Source: CAD feature listing. Evaluate the final solid. Frame: model axes, mm. A direction names the side the tool comes from. Coordinates: 2 decimals unless noted, no trailing zeros. Order: outer loops, then holes, each group sorted by start corner. A loop starts at its lowest first (then second) coordinate and runs counter-clockwise, first axis right, second up. Notation, with made-up numbers: (76, 65.25) -> (83, 65.25) arc R6 ccw to (83, 75.25) -> close; hole circle Ø6 at (-17, 79.5). An arc over 180 degrees is marked (long way). Put each result on its own line as item: value.
from build123d import *

# Parameters (mm, degrees)
EXTRUDE_START            = 8.875
SKETCH1_R                = 7.5
SKETCH1_R_2              = 3
EXTRUDE_KNOB_DEPTH       = 16.5
EXTRUDE_START_2          = 25.375
SKETCH1_3_R              = 3
EXTRUDE_KNOB_INNER_DEPTH = 1
CHAMFER_KNOB_SIZE        = 0.5


with BuildPart() as part:
    # Sketch1 → extrude knob (new body)
    with BuildSketch(Plane.XY.offset(EXTRUDE_START)):
        with Locations((6.776307172, 8.001648034)):
            Circle(SKETCH1_R)
        with Locations((6.776307172, 8.001648034)):
            Circle(SKETCH1_R_2, mode=Mode.SUBTRACT)
    extrude(amount=EXTRUDE_KNOB_DEPTH)

    # Sketch1<3> → extrude knob inner (add)
    with BuildSketch(Plane.XY.offset(EXTRUDE_START_2)):
        with Locations((6.776307172, 8.001648034)):
            Circle(SKETCH1_3_R)
    extrude(amount=-EXTRUDE_KNOB_INNER_DEPTH)

    # chamfer knob
    chamfer_knob_edges = [part.edges().sort_by_distance(p)[0] for p in [
        (-0.723692828, 8.001648034, 25.375),
    ]]
    chamfer(chamfer_knob_edges, length=CHAMFER_KNOB_SIZE)


solid = part.part
1. Set-up query: faces 1 (the flat face through (10, 8, 8.875)), 2 (the cylindrical face through (6.386, 10.976, 16.516)). Return all of +Z, -Z, +X, -X, +Y, -Y with unobstructed straight access to the full face (end or side cutting, diameter ignored); none if empty.
Numbers:
face 1: -Z, +X, -X, +Y, -Y
face 2: -Z
2. First-contact query: pin 1 (6.5 mm diameter, centred on x = 6, y = 7.5, fed in from -Z) (3 decimals); pin 2 (1.5 mm diameter, centred on x = 4, z = 19.5, fed in from +Y); pin 3 (1 mm diameter, centred on x = 8, z = 16.5, fed in from -Y); pin 4 (6 mm diameter, centred on x = 11, z = 13.5, fed in from +Y). Flat tips, straight axial feed; report the tip coordinate or a pass-through.
Numbers:
pin 1: stops at z = 8.875
pin 2: stops at y = 15.22
pin 3: stops at y = 0.54
pin 4: stops at y = 15.4
3. Cut plane A-A on z = 21.5. Output: boundary loops of the cut face in (x, y).
Numbers:
outline: circle Ø15 at (6.78, 8); hole circle Ø6 at (6.78, 8)
4. Pull-direction query (Y, two-part tool) for faces 3 (the flat face through (7, 8, 25.375)), 4 (the flat face through (7, 8, 24.375)), 5 (the cylindrical face through (1.25, 13.07, 16.76)); classes: pulls with the +Y half, pulls with the -Y half, needs draft (parallel to the pull), parting line crosses it, or undercut.
Numbers:
face 3: needs draft
face 4: undercut
face 5: parting line crosses it
5. Ray query, line 1 along X through (y, z) = (7.75, 22.5); line 2 along X through (y, z) = (10.5, 22.5); line 3 along Y through (x, z) = (9.5, 21). Return the intervals inside material, ascending.
Numbers:
line 1: x = -0.72 to 3.79, 9.77 to 14.27
line 2: x = -0.3 to 5.12, 8.44 to 13.85
line 3: y = 1.01 to 6.74, 9.26 to 14.99
